```python
from build123d import *

# Parameters (mm, degrees)
SKETCH_1_W          = 80
SKETCH_1_H          = 50
EXTRUDE_1_DEPTH     = 5
SKETCH_2_W          = 50
SKETCH_2_H          = 50
EXTRUDE_2_DEPTH     = 100
SKETCH_4_W          = 40
SKETCH_4_H          = 42
CUT_EXTRUDE_1_DEPTH = 138.477270849
SKETCH_5_R          = 2.1
CUT_EXTRUDE_2_DEPTH = 10
CUT_EXTRUDE_START   = 10
SKETCH_7_W          = 40
SKETCH_7_H          = 7
CUT_EXTRUDE_7_DEPTH = 128.477270849
EXTRUDE_START       = 44.5
SKETCH_8_W          = 50
SKETCH_8_H          = 15
EXTRUDE_6_DEPTH     = 2.5
SKETCH_9_R          = 1
CUT_EXTRUDE_8_DEPTH = 128.477270849
CHAMFER_2_SIZE      = 4.4
CHAMFER_2_SIZE_2    = 2.540341184
CUT_EXTRUDE_START_2 = 47
SKETCH_14_R         = 5.11141812
CUT_EXTRUDE_9_DEPTH = 91.477270849
CHAMFER_3_SIZE      = 1
CHAMFER_3_SIZE2     = 1.732050808


with BuildPart() as part:
    # 草圖1 → 填料-伸長1 (new body)
    with BuildSketch(Plane.XY):
        with Locations((40, 25)):
            Rectangle(SKETCH_1_W, SKETCH_1_H)
    extrude(amount=EXTRUDE_1_DEPTH)

    # 草圖2 → 填料-伸長2 (add)
    with BuildSketch(Plane.XY):
        with Locations((40, 25)):
            Rectangle(SKETCH_2_W, SKETCH_2_H)
    extrude(amount=EXTRUDE_2_DEPTH)

    # 草圖4 → 除料-伸長1 (cut, through all)
    with BuildSketch(Plane.XY):
        with Locations((40, 26)):
            Rectangle(SKETCH_4_W, SKETCH_4_H)
    extrude(amount=CUT_EXTRUDE_1_DEPTH, mode=Mode.SUBTRACT)

    # 草圖5 → 除料-伸長2 (cut)
    with BuildSketch(Plane.XY):
        with Locations(Location((76.5, 3.5, 0), (0, 0, 180))):
            Circle(SKETCH_5_R)
        with Locations(Location((76.5, 43.5, 0), (0, 0, 180))):
            Circle(SKETCH_5_R)
        with Locations(Location((3.5, 3.5, 0), (0, 0, 180))):
            Circle(SKETCH_5_R)
        with Locations(Location((3.5, 43.5, 0), (0, 0, 180))):
            Circle(SKETCH_5_R)
    extrude(amount=CUT_EXTRUDE_2_DEPTH, mode=Mode.SUBTRACT)

    # 草圖7 → 除料-伸長7 (cut, through all)
    with BuildSketch(Plane(origin=(0, 0, 0), x_dir=(1, 0, 0), z_dir=(0, 1, 0)).offset(CUT_EXTRUDE_START)):
        with Locations((40, -3.5)):
            Rectangle(SKETCH_7_W, SKETCH_7_H)
    extrude(amount=CUT_EXTRUDE_7_DEPTH, mode=Mode.SUBTRACT)

    # 草圖8 → 填料-伸長6 (add)
    with BuildSketch(Plane(origin=(0, 0, 0), x_dir=(1, 0, 0), z_dir=(0, 1, 0)).offset(EXTRUDE_START)):
        with Locations((40, -7.5)):
            Rectangle(SKETCH_8_W, SKETCH_8_H)
    extrude(amount=EXTRUDE_6_DEPTH)

    # 草圖9 → 除料-伸長8 (cut, through all)
    with BuildSketch(Plane(origin=(0, 0, 0), x_dir=(1, 0, 0), z_dir=(0, 1, 0)).offset(CUT_EXTRUDE_START)):
        with Locations(Location((40, -3.5, 0), (0, 0, 270))):
            Circle(SKETCH_9_R)
    extrude(amount=CUT_EXTRUDE_8_DEPTH, mode=Mode.SUBTRACT)

    # 導角2
    # the kernel refuses this chamfer: 4.4, 2.540341184 mm, written as the material it takes off along each edge
    with BuildSketch(Plane(origin=(60, 44.5, 15), x_dir=(0, -0.01932676561270091, -0.9998132206222078), z_dir=(-1, 0, 0))) as chamfer_2_piece_1_section:
        Polygon((CHAMFER_2_SIZE * 0.999813220622, -CHAMFER_2_SIZE * 0.0193267656127), (-CHAMFER_2_SIZE_2 * 0.019326765616, -CHAMFER_2_SIZE_2 * 0.999813220793), (0, 0), align=None)
    chamfer_2_piece_1 = extrude(amount=40, mode=Mode.PRIVATE)
    chamfer_2_piece_1 = split(chamfer_2_piece_1, bisect_by=Plane(origin=(40, 47, 13.532969249), z_dir=(0, -1, 0)), keep=Keep.TOP, mode=Mode.PRIVATE)
    add(chamfer_2_piece_1, mode=Mode.SUBTRACT)

    # 草圖14 → 除料-伸長9 (cut, through all)
    with BuildSketch(Plane(origin=(0, 0, 0), x_dir=(1, 0, 0), z_dir=(0, 1, 0)).offset(CUT_EXTRUDE_START_2)):
        with Locations((40, -6)):
            Circle(SKETCH_14_R)
    extrude(amount=CUT_EXTRUDE_9_DEPTH, mode=Mode.SUBTRACT)

    # 導角3
    chamfer_3_edges = [part.edges().sort_by_distance(p)[0] for p in [
        (40, 50, 11.11141812),
    ]]
    chamfer_3_side = [part.faces().sort_by_distance(p)[0] for p in [
        (40, 50, 51.481645062),
    ]]
    chamfer(chamfer_3_edges, length=CHAMFER_3_SIZE, length2=CHAMFER_3_SIZE2, reference=chamfer_3_side[0])


solid = part.part
```
Source: CAD feature listing. Evaluate the final solid. Frame: model axes, mm. A direction names the side the tool comes from. Give positions to 0.01 mm unless a question says otherwise; leave off trailing zeros. Write each loop counter-clockwise with the first axis right and the second up, starting at its lowest first coordinate (ties: lowest second). Pieces come first, ordered by that corner, then holes.
1. Pull-direction query (Y, two-part tool) for faces 1 (the face through (62, 25, 100)), 2 (the face through (40, 47, 57)), 3 (the face through (39, 50, 49)); classes: +Y half, -Y half, draft (parallel to the pull), parting line (faces both ways), or undercut.
2. Section query A-A (y = 32.5). Return the cut outline in (x, z), then the cut area to 3 significant figures.
3. Access query for faces 4 (the face through (72, 25, 5)), 5 (the face through (40, 5, 49)), 6 (the face through (40.28, 45.73, 12.73)), 7 (the face through (15, 25, 52)), 8 (the face through (39.9, 47.63, 11.11)). Directions: +Z, -Z, +X, -X, +Y, -Y. A direction counts if a zero-diameter tool reaches every point of the face in a straight line with its end or side. Return the directions, or none.
4. Section query C-C (z = 39). Return the cut outline in (x, y), then the cut area to 3 significant figures.
5. First-contact query: pin 1 (5 mm diameter, centred on x = 3.5, y = 43.5, fed in from +Z); pin 2 (10 mm diameter, centred on x = 43, y = 40, fed in from +Z); pin 3 (4 mm diameter, centred on x = 76.5, y = 3.5, fed in from -Z); pin 4 (1 mm diameter, centred on y = 44, z = 65.5, fed in from +X). Flat tips, straight axial feed; report the tip coordinate or a pass-through.
6. Material intervals for line 1 along Y through (x, z) = (3.5, 2.35); line 2 along X through (y, z) = (43.5, 1.95); line 3 along X through (y, z) = (46, 74.5), sorted ascending.
7. Section query D-D (y = 3.5). Return the cut outline in (x, z), then the cut area to 3 significant figures.
8. Section query B-B (x = 3.5). Return the cut outline in (y, z), then the cut area to 3 significant figures.
Output values:
1. face 1: draft
1. face 2: undercut
1. face 3: +Y half
2. outline: (0, 0) - (20, 0) - (20, 100) - (15, 100) - (15, 5) - (0, 5) - close; (60, 0) - (80, 0) - (80, 5) - (65, 5) - (65, 100) - (60, 100) - close
2. area: 1,150 mm2
3. face 4: +Z, +X, +Y, -Y
3. face 5: +Z, -Z
3. face 6: +Z
3. face 7: +Z, -X, +Y, -Y
3. face 8: -Z, +Y
4. outline: (15, 0) - (65, 0) - (65, 50) - (15, 50) - close; hole (20, 5) - (60, 5) - (60, 47) - (20, 47) - close
4. area: 820 mm2
5. pin 1: stops at z = 5
5. pin 2: stops at z = 11.47
5. pin 3: passes through
5. pin 4: stops at x = 65
6. line 1: y = 0 to 1.4, 5.6 to 41.4, 45.6 to 50
6. line 2: x = 0 to 1.4, 5.6 to 20, 60 to 74.4, 78.6 to 80
6. line 3: x = 15 to 20, 60 to 65
7. outline: (0, 0) - (1.4, 0) - (1.4, 5) - (0, 5) - close; (5.6, 0) - (74.4, 0) - (74.4, 5) - (65, 5) - (65, 100) - (15, 100) - (15, 5) - (5.6, 5) - close; (78.6, 0) - (80, 0) - (80, 5) - (78.6, 5) - close
7. area: 5,110 mm2
8. outline: (0, 0) - (1.4, 0) - (1.4, 5) - (0, 5) - close; (5.6, 0) - (41.4, 0) - (41.4, 5) - (5.6, 5) - close; (45.6, 0) - (50, 0) - (50, 5) - (45.6, 5) - close
8. area: 208 mm2
